Autodesk Inventor part; units mm, degrees
ref_plane "YZ Plane" through (0, 0, 0) normal (1, 0, 0) x (0, 1, 0)
ref_plane "XZ Plane" through (0, 0, 0) normal (0, 1, 0) x (-1, 0, 0)
ref_plane "XY Plane" through (0, 0, 0) normal (0, 0, 1) x (1, 0, 0)
sketch "Sketch1" plane through (0, 0, 0) normal (0, 0, 1) x (1, 0, 0)
  line L0 (-25, 25) -> (25, 25)
  line L1 (25, 25) -> (25, -25)
  line L2 (25, -25) -> (-25, -25)
  line L3 (-25, -25) -> (-25, 25)
  line L4 (20, 20) -> (-20, 20)
  line L5 (-20, 20) -> (-20, -20)
  line L6 (-20, -20) -> (20, -20)
  line L7 (20, -20) -> (20, 20)
  point P0 (0, 0)
  dimension "d0" = 50
  dimension "d1" = 50
  dimension "d2" = 25
  dimension "d3" = 25
  dimension "d4" = 5
extrude "Extrusion1" add sketch "Sketch1" along normal blind 700
fillet "Fillet1" radius 2 4 edges at (25, 25, 350) (-25, 25, 350) (25, -25, 350) (-25, -25, 350)
sketch "Sketch2" plane through (-23, 25, 0) normal (0, 1, 0) x (1, 0, 0)
  line L0 (46, 0) -> (0, 0)
  line L1 (46, -700) -> (0, -700)
  point P0 (23, 0)
  point P1 (23, -45)
  point P2 (23, -655)
  dimension "d8" = 45
  dimension "d9" = 0
  dimension "d10" = 45
  dimension "d11" = 0
hole "endHoles" at (0, 25, 45) at (0, 25, 655) direction (0, -1, 0) diameter 10 depth 5
sketch "Sketch3" plane through (25, -23, 0) normal (1, 0, 0) x (0, 0, -1)
  line L0 (0, 23) -> (-550, 23)
  point P0 (-400, 23)
  dimension "d19" = 400
  dimension "d21" = 0
  dimension "d22" = 0
  dimension "d49" = 150
hole "Hole4" at (25, 0, 400) at (25, 0, 550) direction (-1, 0, 0) diameter 10 end through all
equation "\"d0\" = w"
equation "\"d1\" = w"
equation "\"d4\" = t"
equation "\"support_frame_endHoleBuffer\" = 45"
equation "\"d7\" = fillet"
equation "\"d42\" = support_frame_clampHoleDiameter"
equation "\"w\" = support_frame_squareBarDimension"
equation "\"t\" = support_frame_squareBarThickness"
equation "\"fillet\" = support_frame_squareBarFillet"
equation "\"buffer\" = support_frame_endHoleBuffer"
equation "\"hoop_angle_z\" = 45deg"
equation "\"hoop_bearing_length\" = 5deg"
equation "\"hoop_cable_diam\" = 5"
equation "\"hoop_cable_pulley_diam\" = 22"
equation "\"hoop_thickness_large\" = 4"
equation "\"hoop_thickness_medium\" = 3.2"
equation "\"hoop_thickness_small\" = 2"
equation "\"hoop_width_large\" = 51"
equation "\"hoop_width_medium\" = 33.7"
equation "\"hoop_width_small\" = 25.4"
equation "\"rack_tooth_addendum\" = 5"
equation "\"rack_tooth_dedendum\" = 5"
equation "\"rack_tooth_thickness\" = 5"
equation "\"secure_arm_angle\" = 35deg"
equation "\"secure_arm_radii\" = 9"
equation "\"support_baseClamp_platformLengthBuffer\" = 35"
equation "\"support_baseClamp_platformThickness\" = 15"
equation "\"support_baseClamp_platformWidthBuffer\" = 0"
equation "\"support_baseClamp_sleeveHoleDiameter\" = 12"
equation "\"support_baseClamp_sleeveSweepTerminationAngle\" = 55deg"
equation "\"support_baseClamp_thickness\" = 8"
equation "\"support_frame_clampHoleDiameter\" = 10"
equation "\"support_frame_squareBarFillet\" = 2"
equation "\"support_frame_squareBarThickness\" = 5"
equation "\"hoop_tabs_thickness\" = 6"
equation "\"wheelchair_deployed_length\" = 1067"
equation "\"wheelchair_deployed_height\" = 914"
equation "\"hoop_tabs_hole\" = 12"
equation "\"wheelchair_deployed_width\" = 635"
equation "\"sm_varx_pinPlate_thickness\" = 5"
equation "\"sm_varx_member_tolerance\" = 0.5"
equation "\"sm_varx_pinPlate_holeDiameter\" = 5"
equation "\"sm_varx_squareBarThickness\" = 2.5"
equation "\"hoop_bushing23_radialInterference\" = 0"
equation "\"hoop_bushing12_radialInterference\" = 0"
equation "\"hoop_bushing12_od\" = -2 * hoop_thickness_large + hoop_width_large + hoop_bushing12_radialInterference"
equation "\"wheelchatir_pos_deploy_angle_0\" = 65deg"
equation "\"wheelchatir_pos_store_angle_0\" = 90deg"
equation "\"wheelchatir_pos_deploy_angle_1\" = 20deg"
equation "\"wheelchatir_pos_store_angle_1\" = 20deg"
equation "\"hoop_bushing23_od\" = -2 * hoop_thickness_medium + hoop_width_medium + hoop_bushing23_radialInterference"
equation "\"hoop_bushing12_thickness\" = -hoop_width_medium + hoop_bushing12_od - 2 * hoop_bushing12_radialInterference"
equation "\"hoop_bushing23_thickness\" = -hoop_width_small + hoop_bushing23_od - 2 * hoop_bushing23_radialInterference"
properties part number "support_frame_x" material "Steel, Mild"
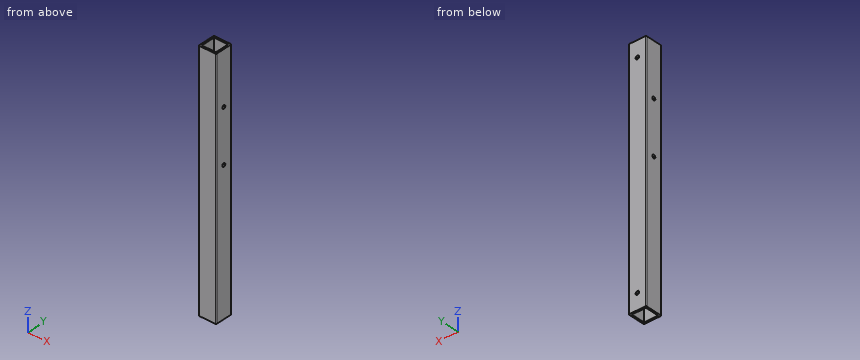
Build history of the part. All positions in model axes, mm. Give positions to 0.01 mm unless a question says otherwise; leave off trailing zeros. Loops run counter-clockwise (first coordinate to the right, second up) from the corner with the lowest first, then second, coordinate; pieces in that order, holes last. Notation, with made-up numbers: (15.25, 67) -> (42.25, 67) arc R36 ccw to (42.25, 105) -> close; hole circle Ø9 at (60.5, 4.25). An arc over 180 degrees is marked (long way). One line per question, with ' | ' between items. Start each with the question number.
1) Cut at A-A (x = -11). Give the cut face in (y, z).
2) Cut at B-B (z = 266). Give the cut face in (x, y), plus the area to 3 significant figures.
3) Probe L1, parallel to Z at x = 21.05, y = 0; L2, parallel to Z at x = 0, y = 23.6; L3, parallel to Y at x = 18, z = 259. List the from-to ranges inside material, lowest first.
Return value:
1) outline: (-25, 0) -> (-20, 0) -> (-20, 700) -> (-25, 700) -> close; (20, 0) -> (25, 0) -> (25, 700) -> (20, 700) -> close
2) outline: (-25, -23) arc R2 ccw to (-23, -25) -> (23, -25) arc R2 ccw to (25, -23) -> (25, 23) arc R2 ccw to (23, 25) -> (-23, 25) arc R2 ccw to (-25, 23) -> close; hole (-20, -20) -> (20, -20) -> (20, 20) -> (-20, 20) -> close | area: 897 mm^2
3) L1: 0 to 395, 405 to 545, 555 to 700 | L2: 0 to 40, 50 to 650, 660 to 700 | L3: -25 to -20, 20 to 25
